from build123d import *

# Parameters (mm, degrees)
SKETCH1_R             = 3.617136877
BOSS_EXTRUDE1_DEPTH   = 40
F_5_0MM_DOWEL_HOLE1_D = 5


with BuildPart() as part:
    # Sketch1 → Boss-Extrude1 (new body)
    with BuildSketch(Plane.XY):
        Polygon((-15, -15), (-4.922326912, -25.077673088), (4.922326912, -25.077673088), (15, -15), (15, 15), (-15, 15), align=None)
        with Locations((0, -18.555652187)):
            Circle(SKETCH1_R, mode=Mode.SUBTRACT)
    extrude(amount=BOSS_EXTRUDE1_DEPTH)

    # Ø5.0mm Dowel Hole1 (through all)
    with Locations(Plane(origin=(15, 8.941860577, 7.42320161), x_dir=(0, 1, 0), z_dir=(1, 0, 0))):
        with Locations((0, 0)):
            Hole(F_5_0MM_DOWEL_HOLE1_D / 2)


solid = part.part
Design review of the part built by this model. Coordinates are the model's own, in mm. Give positions to 0.01 mm unless a question says otherwise; leave off trailing zeros. Order: outer loops, then holes, each group sorted by start corner. A loop starts at its lowest first (then second) coordinate and runs counter-clockwise, first axis right, second up.
1. Add section B-B, the plane x = 0. State the section outline as (y, z) points.
Solution:
outline: (-25.08, 0) - (-22.17, 0) - (-22.17, 40) - (-25.08, 40) - close; (-14.94, 0) - (15, 0) - (15, 40) - (-14.94, 40) - close; hole circle Ø5 at (8.94, 7.42)
2. For pin 1 Ø5 at (x, y) = (2, 11) entering from -Z; pin 2 Ø12 at (x, z) = (11.5, 15) entering from -Y, all flat-tipped, find the tip position at first contact; note any pin that passes through.
Solution:
pin 1: stops at z = 0
pin 2: stops at y = -24.5
3. Add section A-A, the plane z = 9. State the section outline as (x, y) points, then the cut area to 3 significant figures.
Solution:
outline: (-15, -15) - (-4.92, -25.08) - (4.92, -25.08) - (15, -15) - (15, 7) - (-15, 7) - close; (-15, 10.88) - (15, 10.88) - (15, 15) - (-15, 15) - close; hole circle Ø7.23 at (0, -18.56)
area: 943 mm2
4. Add section C-C, the plane z = 31.5. State the section outline as (x, y) points.
Solution:
outline: (-15, -15) - (-4.92, -25.08) - (4.92, -25.08) - (15, -15) - (15, 15) - (-15, 15) - close; hole circle Ø7.23 at (0, -18.56)
5. Mouldability with a two-part tool opening along Y and no side actions: class faces 1 (the flat face through (-15, 0, 20)), 2 (the cylindrical face through (-0.21, 7.598, 9.531)), 3 (the flat face through (0, -25.078, 20)) as +Y half, -Y half, draft (parallel to the pull), parting line (faces both ways), or undercut.
Solution:
face 1: draft
face 2: undercut
face 3: -Y half
6. To check wall thickness, follow L1, parallel to Y at x = 0, z = 31; L2, parallel to X at y = -19, z = 38; L3, parallel to Z at x = 12, y = 9. State the ranges of each line that lie inside material, in increasing order.
Solution:
L1: y = -25.08 to -22.17, -14.94 to 15
L2: x = -11 to -3.59, 3.59 to 11
L3: z = 0 to 4.92, 9.92 to 40
7. Add section D-D, the plane x = -6. State the section outline as (y, z) points, then the cut area to 3 significant figures.
Solution:
outline: (-24, 0) - (15, 0) - (15, 40) - (-24, 40) - close; hole circle Ø5 at (8.94, 7.42)
area: 1,540 mm2
